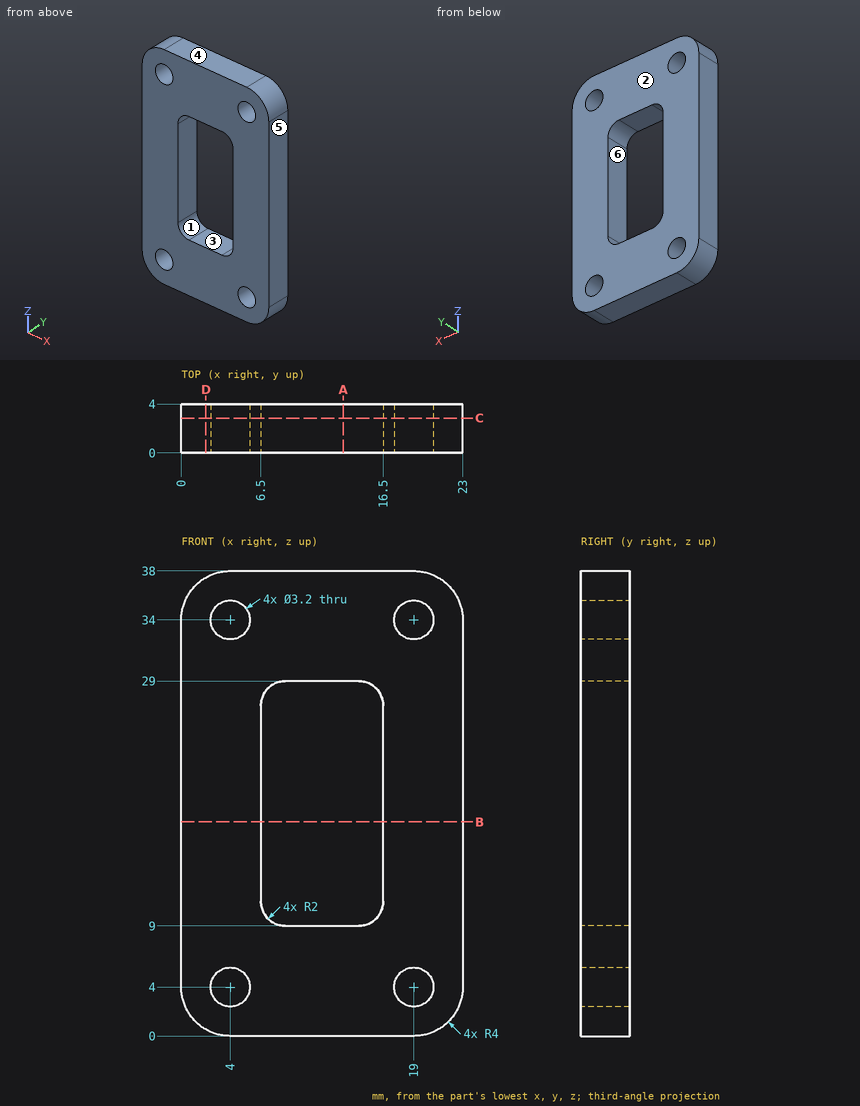
The drawing under review shows one solid part. Ordinate dimensions are in mm from its lowest x, y, z. A direction names the side the tool comes from. Round coordinates to 2 decimals unless told otherwise and drop trailing zeros. Loops run counter-clockwise (first coordinate to the right, second up) from the corner with the lowest first, then second, coordinate; pieces in that order, holes last. Notation, with made-up numbers: (17.25, 68.25) -> (66.25, 68.25) arc R29 ccw to (66.25, 89.25) -> close; hole circle Ø6 at (86, 72.5). An arc over 180 degrees is marked (long way). One line per question, with ' | ' between items. Start each with the question number.
Item 1: Wall thickness on line 1 along X through (y, z) = (1.4, 34); line 2 along X through (y, z) = (2.7, 13.5); line 3 along X through (y, z) = (3.8, 3.5): over which ranges is each line inside the solid? List them lowest first. Write a range as [from, to].
Item 2: Add section B-B, the plane z = 17.5. Write out the cut boundary in (x, y).
Item 3: Add section A-A, the plane x = 13.25. Write out the cut boundary in (y, z).
Item 4: Machinability: for the marked faces 1 and 2, which of the approach directions +Z, -Z, +X, -X, +Y, -Y give a long, thin tool a straight path to every point of the face, cutting with its end or side? Answer none if there is none.
Item 5: Draft analysis for pull direction Z (two halves, no side actions). For the marked faces 3, 4, 5 and 6, state which applies: +Z half, -Z half, draft (parallel to the pull), parting line (faces both ways), or undercut.
Item 6: For pin 1 (2 mm diameter, centred on x = 2.5, y = 2, fed in from +Z); pin 2 (1.5 mm diameter, centred on y = 0.5, z = 24.5, fed in from -X), all flat-tipped, find the tip position at first contact; note any pin that passes through.
Item 7: Add section C-C, the plane y = 2.85. Write out the cut boundary in (x, z), then the cut area to 3 significant figures.
Item 8: Add section D-D, the plane x = 2. Write out the cut boundary in (y, z), then the cut area to 3 significant figures.
Return value:
1) line 1: x = [0, 2.4], [5.6, 17.4], [20.6, 23] | line 2: x = [0, 6.5], [16.5, 23] | line 3: x = [0.03, 2.48], [5.52, 17.48], [20.52, 22.97]
2) outline: (0, 0) -> (6.5, 0) -> (6.5, 4) -> (0, 4) -> close; (16.5, 0) -> (23, 0) -> (23, 4) -> (16.5, 4) -> close
3) outline: (0, 0) -> (4, 0) -> (4, 9) -> (0, 9) -> close; (0, 29) -> (4, 29) -> (4, 38) -> (0, 38) -> close
4) face 1: +Y, -Y | face 2: +Z, -Z, +X, -X, +Y
5) face 3: undercut | face 4: +Z half | face 5: draft | face 6: undercut
6) pin 1: stops at z = 37.97 | pin 2: stops at x = 0
7) outline: (0, 4) arc R4 ccw to (4, 0) -> (19, 0) arc R4 ccw to (23, 4) -> (23, 34) arc R4 ccw to (19, 38) -> (4, 38) arc R4 ccw to (0, 34) -> close; hole circle Ø3.2 at (4, 4); hole circle Ø3.2 at (4, 34); hole (6.5, 11) arc R2 ccw to (8.5, 9) -> (14.5, 9) arc R2 ccw to (16.5, 11) -> (16.5, 27) arc R2 ccw to (14.5, 29) -> (8.5, 29) arc R2 ccw to (6.5, 27) -> close; hole circle Ø3.2 at (19, 4); hole circle Ø3.2 at (19, 34) | area: 632 mm2
8) outline: (0, 0.54) -> (4, 0.54) -> (4, 37.46) -> (0, 37.46) -> close | area: 148 mm2
